The listing builds one solid part. Answer for the finished solid, in the listing's coordinates (mm). A direction names the side the tool comes from. Coordinates: 2 decimals unless noted, no trailing zeros. Write each loop counter-clockwise with the first axis right and the second up, starting at its lowest first coordinate (ties: lowest second). Pieces come first, ordered by that corner, then holes.
```python
from build123d import *

# Parameters (mm, degrees)
F0_R     = 90.059663
F1_DEPTH = 6
F3_DEPTH = 80


with BuildPart() as f1:
    # F0 (on Top) → F1 (new body)
    with BuildSketch(Plane.XY):
        Circle(F0_R)
    extrude(amount=F1_DEPTH)

    # F2 (on face) → F3 (join)
    with BuildSketch(Plane.XY.offset(6)):
        Polygon((41.894139, 67.897459), (37.471054, 70.256495), (3.045908, 5.710936), align=None)
        Polygon((75.548055, -13.42053), (6.37266, -1.132054), (74.672942, -18.346794), align=None)
        Polygon((9.701488, -75.674326), (0, -6), (3.045908, -76.601053), align=None)
        Polygon((-54.17126, 58.228912), (-3.056724, 5.162987), (-50.558788, 61.708542), align=None)
        Polygon((-65.313227, -32.813866), (-4.909957, -3.448525), (-67.902333, -27.488185), align=None)
    extrude(amount=F3_DEPTH)


solid = f1.part
```
(1) Section D-D, the plane y = -73 is taken. Write down the section's boundary in (x, z), plus the area to 3 significant figures.
(2) Section C-C, the plane x = 29 is taken. Write down the section's boundary in (y, z), plus the area to 3 significant figures.
(3) Each of these flat-tipped pins is pushed along its axis until it touches: pin 1 (12 mm diameter, centred on y = -37, z = 38, fed in from +X); pin 2 (12 mm diameter, centred on x = -70, y = -46.5, fed in from +Z); pin 3 (4 mm diameter, centred on x = 50.5, z = 73.5, fed in from +Y). Where does it stop, or does it pass through?
(4) Section A-A, the plane z = 49.5 is taken. Write down the section's boundary in (x, y).
(5) Which of the six approach directions +Z, -Z, +X, -X, +Y, -Y give full straight-line access (tool end or side, diameter ignored) to faces 1 (the flat face through (-66.626, -30.114, 45.44)), 2 (the flat face through (4.919, -41.325, 45.44)), 3 (the flat face through (41.44, -7.36, 45.44)), 4 (the flat face through (39.714, 69.06, 45.44))?
(6) Find the intervals of material crossed by probe 1 along X at (y, z) = (59.5, 13); probe 2 along Z at (x, y) = (-45.5, 4); probe 3 along X at (y, z) = (33, 32.5), in increasing order.
(7) Section B-B, the plane y = -37 is taken. Write down the section's boundary in (x, z), plus the area to 3 significant figures.
(8) For a pull along Y with two mould halves and no side action, classify faces 5 (the flat face through (6.327, -76.144, 45.44)), 6 (the flat face through (22.2, 36.37, 45.44)), 7 (the flat face through (-26.475, 33.04, 45.44)) as pulls with the +Y half, pulls with the -Y half, needs draft (parallel to the pull), parting line crosses it, or undercut.
Solution:
1. outline: (-52.74, 0) - (52.74, 0) - (52.74, 6) - (9.33, 6) - (9.33, 86) - (2.89, 86) - (2.89, 6) - (-52.74, 6) - close
1. area: 1,150 mm2
2. outline: (-85.26, 0) - (85.26, 0) - (85.26, 6) - (54.37, 6) - (54.37, 86) - (47.26, 86) - (47.26, 6) - (-5.15, 6) - (-5.15, 86) - (-6.84, 86) - (-6.84, 6) - (-85.26, 6) - close
2. area: 1,730 mm2
3. pin 1: stops at x = 5.15
3. pin 2: stops at z = 6
3. pin 3: stops at y = -8.62
4. outline: (-67.9, -27.49) - (-65.31, -32.81) - (-4.91, -3.45) - close; (-54.17, 58.23) - (-3.06, 5.16) - (-50.56, 61.71) - close; (0, -6) - (3.05, -76.6) - (9.7, -75.67) - close; (3.05, 5.71) - (41.89, 67.9) - (37.47, 70.26) - close; (6.37, -1.13) - (74.67, -18.35) - (75.55, -13.42) - close
5. face 1: +Z, -X, -Y
5. face 2: +Z
5. face 3: +Z, +X
5. face 4: +Z, +X, +Y
6. probe 1: x = -52.85 to -48.7, 31.73 to 36.65
6. probe 2: z = 0 to 6
6. probe 3: x = -29.87 to -26.44, 17.6 to 20.09
7. outline: (-82.11, 0) - (82.11, 0) - (82.11, 6) - (4.32, 6) - (4.32, 86) - (1.34, 86) - (1.34, 6) - (-82.11, 6) - close
7. area: 1,220 mm2
8. face 5: pulls with the -Y half
8. face 6: undercut
8. face 7: pulls with the +Y half
